from build123d import *

# Parameters (mm, degrees)
SKETCH_1_R          = 75
EXTRUDE_1_DEPTH     = 50
SKETCH_3_R          = 50
SKETCH_2_R          = 75
FILLET_1_R          = 10
SKETCH_4_R          = 10
CUT_EXTRUDE_1_DEPTH = 140.104278635
SHELL_1_T           = -3


with BuildPart() as part:
    # 草图1 → 凸台-拉伸1 (new body)
    with BuildSketch(Plane.XY):
        Circle(SKETCH_1_R)
    extrude(amount=EXTRUDE_1_DEPTH)

    # 草图3 → 放样1 section 0
    with BuildSketch(Plane(origin=(0, 0, -40), x_dir=(-1, 0, 0), z_dir=(0, 0, -1))):
        Circle(SKETCH_3_R)
    # 草图2 → 放样1 section 1
    with BuildSketch(Plane(origin=(0, 0, 0), x_dir=(-1, 0, 0), z_dir=(0, 0, -1))):
        Circle(SKETCH_2_R)
    loft()

    # 圆角1
    fillet_1_edges = [part.edges().sort_by_distance(p)[0] for p in [
        (50, 0, -40),
        (0, 75, 0),
    ]]
    fillet(fillet_1_edges, radius=FILLET_1_R)

    # 草图4 → 切除-拉伸1 (cut, through all)
    with BuildSketch(Plane(origin=(0, 0, -40), x_dir=(-1, 0, 0), z_dir=(0, 0, -1))):
        Circle(SKETCH_4_R)
    extrude(amount=-CUT_EXTRUDE_1_DEPTH, mode=Mode.SUBTRACT)

    # 抽壳1
    shell_1_openings = [part.faces().sort_by_distance(p)[0] for p in [
        (10, 0, 5),
    ]]
    offset(amount=SHELL_1_T, openings=shell_1_openings, kind=Kind.INTERSECTION)


solid = part.part
Design review of the part built by this model. Coordinates are the model's own, in mm. A direction names the side the tool comes from. Give positions to 0.01 mm unless a question says otherwise; leave off trailing zeros. Write each loop counter-clockwise with the first axis right and the second up, starting at its lowest first coordinate (ties: lowest second). Pieces come first, ordered by that corner, then holes. Notation, with made-up numbers: M 47.25,-39 L 89.25,-39 A24 ccw 89.25,-9 Z; hole C 38.5,43.5 d1. An arc over 180 degrees is marked long. Answer as a JSON object with one key per item and string values. Group by question number.
1) For line 1 along Z through (x, y) = (-23.5, -14.5); line 2 along Y through (x, z) = (0, 31); line 3 along Y through (x, z) = (0, 47.75), list the stretches that pass through material, from the lowest coordinate up.
2) We need section A-A (z = 16.5). Give the boundary of the cut face in (x, y).
3) Clearance check with flat-ended pins moving along their axes: pin 1 Ø10 at (x, z) = (13, 8) entering from -Y; pin 2 Ø1.5 at (y, z) = (13.5, -25.5) entering from -X; pin 3 Ø3 at (x, z) = (53.5, -15.5) entering from +Y; pin 4 Ø18 at (x, y) = (0, 0) entering from +Z. State where each tip first meets the part, or that it passes through.
4) Tool access review of faces 1 (the face through (-1, -15, 47)), 2 (the face through (7.059, 53.761, -33.244)): name each direction out of +Z, -Z, +X, -X, +Y, -Y from which nothing blocks a thin tool from reaching the whole face with its end or side.
5) Mouldability with a two-part tool opening along Y and no side actions: class faces 3 (the face through (11, 1, -40)), 4 (the face through (11, 1, -37)), 5 (the face through (-9.764, 74.362, 26.104)) as released by +Y, released by -Y, zero draft, split by the parting line, or undercut.
Answer key:
{
 "1": {"line 1": "z = -40 to -37, 47 to 50", "line 2": "y = -75 to -72, 72 to 75", "line 3": "y = -75 to -10, 10 to 75"},
 "2": {"outline": "C 0,0 d150; hole C 0,0 d144"},
 "3": {"pin 1": "stops at y = -74.57", "pin 2": "stops at x = -58.01", "pin 3": "stops at y = 40.05", "pin 4": "passes through"},
 "4": {"face 1": "none", "face 2": "-Z"},
 "5": {"face 3": "zero draft", "face 4": "undercut", "face 5": "split by the parting line"}
}
